```python
from build123d import *

# Parameters (mm, degrees)
SKETCH1_R           = 8
BOSS_EXTRUDE1_DEPTH = 25
CUT_EXTRUDE1_DEPTH  = 10


with BuildPart() as part:
    # Sketch1 → Boss-Extrude1 (new body)
    with BuildSketch(Plane(origin=(0, 0, 0), x_dir=(1, 0, 0), z_dir=(0, 1, 0))):
        with Locations(Location((0, 0, 0), (0, 0, 270))):
            Circle(SKETCH1_R)
        with BuildLine():
            ThreePointArc((-3.098386677, 2.2), (0, -3.8), (3.098386677, 2.2))
            Line((3.098386677, 2.2), (-3.098386677, 2.2))
        make_face(mode=Mode.SUBTRACT)
    extrude(amount=BOSS_EXTRUDE1_DEPTH)

    # Sketch2 → Cut-Extrude1 (cut)
    with BuildSketch(Plane.XZ):
        with BuildLine():
            Line((-2.645751311, -3), (2.645751311, -3))
            ThreePointArc((2.645751311, -3), (0, 4), (-2.645751311, -3))
        make_face()
    extrude(amount=-CUT_EXTRUDE1_DEPTH, mode=Mode.SUBTRACT)


solid = part.part
```
Here's how the part is built. I have some questions about the finished solid (model axes, mm). A direction names the side the tool comes from. Coordinates: 2 decimals unless noted, no trailing zeros. Order: outer loops, then holes, each group sorted by start corner. A loop starts at its lowest first (then second) coordinate and runs counter-clockwise, first axis right, second up.
1) Imagine slicing it at B-B on z = 0. List the corners of the cut face in (x, y) for me.
2) Which directions (+Z, -Z, +X, -X, +Y, -Y) give clear straight access to the entire face, cutting with the end or side of a thin tool? Please do faces 5 (the face through (0, 5, 4)), 6 (the face through (0, 0, -4)).
3) Imagine slicing it at A-A on x = 0. List the corners of the cut face in (y, z) for me.
4) We'd pull the mould along X, two halves only. Please class faces 1 (the face through (0, 25, -4)), 2 (the face through (0, 5, -3)), 3 (the face through (-7.81, 12.32, -1.73)), 4 (the face through (0, 17, -2.2)): +X half, -X half, draft (parallel to the pull), parting line (faces both ways), or undercut.
5) Will these pins go through, and if not, where does the flat tip stop? pin 1 (1.5 mm diameter, centred on x = -6, y = 3, fed in from +Z); pin 2 (2 mm diameter, centred on y = 3, z = 1.5, fed in from +X); pin 3 (6 mm diameter, centred on y = 6, z = -5, fed in from +X).
6) Imagine slicing it at C-C on y = 17. List the corners of the cut face in (x, z) for me, and give its area (3 significant figures).
7) Imagine slicing it at D-D on z = 4.5. List the corners of the cut face in (x, y) for me, and give its area (3 significant figures).
8) I need wall thicknesses on line 1 (X direction, y = 20.5, z = 0); line 2 (X direction, y = 6, z = 0); line 3 (Z direction, x = -3, y = 2). Which ranges of each line are inside material? Lowest first, please.
Response values:
1. outline: (-8, 0) - (-4, 0) - (-4, 10) - (-3.8, 10) - (-3.8, 25) - (-8, 25) - close; (3.8, 10) - (4, 10) - (4, 0) - (8, 0) - (8, 25) - (3.8, 25) - close
2. face 5: -Y
2. face 6: +Z, -Z, +X, -X, -Y
3. outline: (0, -8) - (25, -8) - (25, -2.2) - (10, -2.2) - (10, -3) - (0, -3) - close; (0, 4) - (10, 4) - (10, 3.8) - (25, 3.8) - (25, 8) - (0, 8) - close
4. face 1: draft
4. face 2: undercut
4. face 3: parting line
4. face 4: undercut
5. pin 1: stops at z = 6.04
5. pin 2: stops at x = 7.98
5. pin 3: stops at x = 7.75
6. outline: circle Ø16 at (0, 0); hole (-3.1, -2.2) - (3.1, -2.2) arc R3.8 ccw (long way) to start
6. area: 163 mm2
7. outline: (-6.61, 0) - (6.61, 0) - (6.61, 25) - (-6.61, 25) - close
7. area: 331 mm2
8. line 1: x = -8 to -3.8, 3.8 to 8
8. line 2: x = -8 to -4, 4 to 8
8. line 3: z = -7.42 to -2.65, 2.65 to 7.42
